```python
from build123d import *

# Parameters (mm, degrees)
SKETCH1_W           = 39.9161
SKETCH1_H           = 36.1569
BOSS_EXTRUDE1_DEPTH = 19.812
SKETCH2_W           = 2.4892
SKETCH2_H           = 18.923
BOSS_EXTRUDE3_DEPTH = 6.4389
SKETCH4_W           = 2.54
SKETCH4_H           = 18.923
BOSS_EXTRUDE4_DEPTH = 6.4389
SKETCH5_R           = 2.8829
BOSS_EXTRUDE5_DEPTH = 2.54


with BuildPart() as part:
    # Sketch1 → Boss-Extrude1 (new body)
    with BuildSketch(Plane(origin=(0, 0, 0), x_dir=(1, 0, 0), z_dir=(0, 1, 0))):
        with Locations((-19.95805, -18.07845)):
            Rectangle(SKETCH1_W, SKETCH1_H)
    extrude(amount=BOSS_EXTRUDE1_DEPTH)

    # Sketch2 → Boss-Extrude3 (add)
    with BuildSketch(Plane(origin=(0, 0, 0), x_dir=(0, 0, -1), z_dir=(1, 0, 0))):
        with Locations((-27.7241, 9.8171)):
            Rectangle(SKETCH2_W, SKETCH2_H)
    extrude(amount=BOSS_EXTRUDE3_DEPTH)

    # Sketch4 → Boss-Extrude4 (add)
    with BuildSketch(Plane.ZY.offset(39.9161)):
        with Locations((27.813, 10.0457)):
            Rectangle(SKETCH4_W, SKETCH4_H)
    extrude(amount=BOSS_EXTRUDE4_DEPTH)

    # Sketch5 → Boss-Extrude5 (add)
    with BuildSketch(Plane.XY.offset(36.1569)):
        with Locations((-30.3022, 9.906)):
            Circle(SKETCH5_R)
    extrude(amount=BOSS_EXTRUDE5_DEPTH)


solid = part.part
```
Design review of the part built by this model. Coordinates are the model's own, in mm. A direction names the side the tool comes from. Coordinates: 2 decimals unless noted, no trailing zeros. Loops run counter-clockwise (first coordinate to the right, second up) from the corner with the lowest first, then second, coordinate; pieces in that order, holes last.
Q1. We need section B-B on x = -6.5. State the section outline as (y, z) points.
Reported:
outline: (0, 0) - (19.81, 0) - (19.81, 36.16) - (0, 36.16) - close
Q2. Tool access review of faces 1 (the face through (-43, 0.584, 28)), 2 (the face through (-43, 10, 29.083)), 3 (the face through (3, 10, 28.969)), 4 (the face through (3, 0.356, 28)): name each direction out of +Z, -Z, +X, -X, +Y, -Y from which nothing blocks a thin tool from reaching the whole face with its end or side.
Reported:
face 1: +Z, -Z, -X, -Y
face 2: +Z, -X, +Y, -Y
face 3: +Z, +X, +Y, -Y
face 4: +Z, -Z, +X, -Y
Q3. We need section A-A on y = 14. State the section outline as (x, z) points (1 decimal).
Reported:
outline: (-46.4, 26.5) - (-39.9, 26.5) - (-39.9, 0) - (0, 0) - (0, 26.5) - (6.4, 26.5) - (6.4, 29) - (0, 29) - (0, 36.2) - (-39.9, 36.2) - (-39.9, 29.1) - (-46.4, 29.1) - close
Q4. To check wall thickness, follow line 1 (Z direction, x = -21, y = 2.25); line 2 (X direction, y = 9, z = 5.5). State the ranges of each line that lie inside material, in increasing order.
Reported:
line 1: z = 0 to 36.16
line 2: x = -39.92 to 0
Q5. For pin 1 (5 mm diameter, centred on x = -42.5, y = 11, fed in from -Z); pin 2 (6 mm diameter, centred on x = -15.5, y = 14.5, fed in from +Z); pin 3 (1.3 mm diameter, centred on x = -44, z = 28, fed in from +Y), all flat-tipped, find the tip position at first contact; note any pin that passes through.
Reported:
pin 1: stops at z = 26.54
pin 2: stops at z = 36.16
pin 3: stops at y = 19.51
Q6. We need section D-D on y = 9.25. State the section outline as (x, z) points (1 decimal), and give its area (3 significant figures).
Reported:
outline: (-46.4, 26.5) - (-39.9, 26.5) - (-39.9, 0) - (0, 0) - (0, 26.5) - (6.4, 26.5) - (6.4, 29) - (0, 29) - (0, 36.2) - (-27.5, 36.2) - (-27.5, 38.7) - (-33.1, 38.7) - (-33.1, 36.2) - (-39.9, 36.2) - (-39.9, 29.1) - (-46.4, 29.1) - close
area: 1,490 mm2
Q7. We need section C-C on z = 4. State the section outline as (x, y) points.
Reported:
outline: (-39.92, 0) - (0, 0) - (0, 19.81) - (-39.92, 19.81) - close
